from build123d import *

# Parameters (mm, degrees)
SKETCH_1_W      = 560
SKETCH_1_H      = 25
EXTRUDE_1_DEPTH = 2.3


with BuildPart() as part:
    # ｽｹｯﾁ1 → ﾎﾞｽ - 押し出し1 (new body)
    with BuildSketch(Plane.XY):
        with Locations((0, 12.664243194)):
            Rectangle(SKETCH_1_W, SKETCH_1_H)
        with BuildLine():
            Line((-270, 16.381792792), (-244, 16.381792792))
            ThreePointArc((-244, 16.381792792), (-240.5, 12.881792792), (-244, 9.381792792))
            Line((-244, 9.381792792), (-270, 9.381792792))
            ThreePointArc((-270, 9.381792792), (-273.5, 12.881792792), (-270, 16.381792792))
        make_face(mode=Mode.SUBTRACT)
        with BuildLine():
            Line((-230.5, 16.381792792), (-204.5, 16.381792792))
            ThreePointArc((-204.5, 16.381792792), (-201, 12.881792792), (-204.5, 9.381792792))
            Line((-204.5, 9.381792792), (-230.5, 9.381792792))
            ThreePointArc((-230.5, 9.381792792), (-234, 12.881792792), (-230.5, 16.381792792))
        make_face(mode=Mode.SUBTRACT)
        with BuildLine():
            Line((-191, 16.381792792), (-165, 16.381792792))
            ThreePointArc((-165, 16.381792792), (-161.5, 12.881792792), (-165, 9.381792792))
            Line((-165, 9.381792792), (-191, 9.381792792))
            ThreePointArc((-191, 9.381792792), (-194.5, 12.881792792), (-191, 16.381792792))
        make_face(mode=Mode.SUBTRACT)
        with BuildLine():
            Line((-151.5, 16.381792792), (-125.5, 16.381792792))
            ThreePointArc((-125.5, 16.381792792), (-122, 12.881792792), (-125.5, 9.381792792))
            Line((-125.5, 9.381792792), (-151.5, 9.381792792))
            ThreePointArc((-151.5, 9.381792792), (-155, 12.881792792), (-151.5, 16.381792792))
        make_face(mode=Mode.SUBTRACT)
        with BuildLine():
            Line((-112, 16.381792792), (-86, 16.381792792))
            ThreePointArc((-86, 16.381792792), (-82.5, 12.881792792), (-86, 9.381792792))
            Line((-86, 9.381792792), (-112, 9.381792792))
            ThreePointArc((-112, 9.381792792), (-115.5, 12.881792792), (-112, 16.381792792))
        make_face(mode=Mode.SUBTRACT)
        with BuildLine():
            Line((-72.5, 16.381792792), (-46.5, 16.381792792))
            ThreePointArc((-46.5, 16.381792792), (-43, 12.881792792), (-46.5, 9.381792792))
            Line((-46.5, 9.381792792), (-72.5, 9.381792792))
            ThreePointArc((-72.5, 9.381792792), (-76, 12.881792792), (-72.5, 16.381792792))
        make_face(mode=Mode.SUBTRACT)
        with BuildLine():
            Line((-33, 16.381792792), (-7, 16.381792792))
            ThreePointArc((-7, 16.381792792), (-3.5, 12.881792792), (-7, 9.381792792))
            Line((-7, 9.381792792), (-33, 9.381792792))
            ThreePointArc((-33, 9.381792792), (-36.5, 12.881792792), (-33, 16.381792792))
        make_face(mode=Mode.SUBTRACT)
        with BuildLine():
            Line((6.5, 16.381792792), (32.5, 16.381792792))
            ThreePointArc((32.5, 16.381792792), (36, 12.881792792), (32.5, 9.381792792))
            Line((32.5, 9.381792792), (6.5, 9.381792792))
            ThreePointArc((6.5, 9.381792792), (3, 12.881792792), (6.5, 16.381792792))
        make_face(mode=Mode.SUBTRACT)
        with BuildLine():
            Line((46, 16.381792792), (72, 16.381792792))
            ThreePointArc((72, 16.381792792), (75.5, 12.881792792), (72, 9.381792792))
            Line((72, 9.381792792), (46, 9.381792792))
            ThreePointArc((46, 9.381792792), (42.5, 12.881792792), (46, 16.381792792))
        make_face(mode=Mode.SUBTRACT)
        with BuildLine():
            Line((85.5, 16.381792792), (111.5, 16.381792792))
            ThreePointArc((111.5, 16.381792792), (115, 12.881792792), (111.5, 9.381792792))
            Line((111.5, 9.381792792), (85.5, 9.381792792))
            ThreePointArc((85.5, 9.381792792), (82, 12.881792792), (85.5, 16.381792792))
        make_face(mode=Mode.SUBTRACT)
        with BuildLine():
            Line((125, 16.381792792), (151, 16.381792792))
            ThreePointArc((151, 16.381792792), (154.5, 12.881792792), (151, 9.381792792))
            Line((151, 9.381792792), (125, 9.381792792))
            ThreePointArc((125, 9.381792792), (121.5, 12.881792792), (125, 16.381792792))
        make_face(mode=Mode.SUBTRACT)
        with BuildLine():
            Line((164.5, 16.381792792), (190.5, 16.381792792))
            ThreePointArc((190.5, 16.381792792), (194, 12.881792792), (190.5, 9.381792792))
            Line((190.5, 9.381792792), (164.5, 9.381792792))
            ThreePointArc((164.5, 9.381792792), (161, 12.881792792), (164.5, 16.381792792))
        make_face(mode=Mode.SUBTRACT)
        with BuildLine():
            Line((204, 16.381792792), (230, 16.381792792))
            ThreePointArc((230, 16.381792792), (233.5, 12.881792792), (230, 9.381792792))
            Line((230, 9.381792792), (204, 9.381792792))
            ThreePointArc((204, 9.381792792), (200.5, 12.881792792), (204, 16.381792792))
        make_face(mode=Mode.SUBTRACT)
        with BuildLine():
            Line((243.5, 16.381792792), (269.5, 16.381792792))
            ThreePointArc((269.5, 16.381792792), (273, 12.881792792), (269.5, 9.381792792))
            Line((269.5, 9.381792792), (243.5, 9.381792792))
            ThreePointArc((243.5, 9.381792792), (240, 12.881792792), (243.5, 16.381792792))
        make_face(mode=Mode.SUBTRACT)
    extrude(amount=EXTRUDE_1_DEPTH)


solid = part.part
Model file for the job. Use its own axes, mm. Give positions to 0.01 mm unless a question says otherwise; leave off trailing zeros. Loops run counter-clockwise (first coordinate to the right, second up) from the corner with the lowest first, then second, coordinate; pieces in that order, holes last.
Item 1: Slice it at A-A (x = -137). Write the cut outline in (y, z).
Check values:
outline: (0.16, 0) - (9.38, 0) - (9.38, 2.3) - (0.16, 2.3) - close; (16.38, 0) - (25.16, 0) - (25.16, 2.3) - (16.38, 2.3) - close
Item 2: Slice it at B-B (z = 1.1). Give the number of separate pieces and of enclosed holes in the cut face, plus the area to 3 significant figures.
Check values:
separate pieces: 1
enclosed holes: 14
area: 10,900 mm2
Item 3: Drill centre lines: line 1 along Y through (x, z) = (-47, 2.2); line 2 along Y through (x, z) = (-241.5, 0.9). Where is each one in solid material? Low to high.
Check values:
line 1: y = 0.16 to 9.38, 16.38 to 25.16
line 2: y = 0.16 to 10.43, 15.33 to 25.16
